Autodesk Fusion 360 part; units mm, degrees
sketch "Sketch1" plane through (0, 0, 0) normal (0, 1, 0) x (1, 0, 0)
  circle A0 centre (0, 0) radius 45
  dimension "d1" = 90
extrude "Extrude1" add sketch "Sketch1" along normal blind 70 draft -15
sketch "Sketch2" plane through (0, 0, 0) normal (0, 1, 0) x (1, 0, 0)
  circle A0 centre (0, 0) radius 42
  dimension "d4" = 84
extrude "Extrude2" cut sketch "Sketch2" along normal blind 70 draft -15
extrude "Extrude3" add 1 faces at (25.1459, 70, 1.3038) along direction (0, 1, 0) blind 35
Verification items for the finished model (mm, model axes). Coordinates: 2 decimals unless noted, no trailing zeros. Order: outer loops, then holes, each group sorted by start corner. A loop starts at its lowest first (then second) coordinate and runs counter-clockwise, first axis right, second up. Notation, with made-up numbers: (67, -24.75) -> (115, -24.75) arc R17 cw to (115, -15.75) -> close; hole circle Ø1 at (20.5, 49). An arc over 180 degrees is marked (long way). Put each result on its own line as item: value. Start each with the question number.
1. Material ranges on L1, parallel to X at y = 85, z = 0; L2, parallel to Z at x = -9, y = 56.5, recorded low to high. Write a range as [from, to].
2. Cross-section at C-C, the plane y = 75. Record the boundary of the cut face in (x, z), then the cut area to 3 significant figures.
3. Cross-section at D-D, the plane y = 25. Record the boundary of the cut face in (x, z).
4. Mould release check, pull along X, two halves, no side actions. Record for faces 1 (the cylindrical face through (-3.42, 87.26, 26.02)), 2 (the conical face through (29.253, 42.288, 9.212)), 3 (the flat face through (-15.7, 105, 17.4)): released by +X, released by -X, zero draft, split by the parting line, or undercut.
5. Cross-section at B-B, the plane x = 0. Record the boundary of the cut face in (y, z).
6. Go/stop test with flat-tipped pins: pin 1 Ø4 at (y, z) = (75, -2.5) entering from -X; pin 2 Ø5 at (x, y) = (33.5, 22.5) entering from +Z; pin 3 Ø3 at (x, y) = (22, 57.5) entering from +Z. Record where each tip stops, or that it passes through.
7. Cross-section at A-A, the plane z = 0. Record the boundary of the cut face in (x, y), then the cut area to 3 significant figures.
Computed:
1. L1: [-26.24, -23.24], [23.24, 26.24]
1. L2: [-28.47, -25.31], [25.31, 28.47]
2. outline: circle Ø52.49 at (0, 0); hole circle Ø46.49 at (0, 0)
2. area: 466 mm2
3. outline: circle Ø76.6 at (0, 0); hole circle Ø70.6 at (0, 0)
4. face 1: split by the parting line
4. face 2: undercut
4. face 3: zero draft
5. outline: (0, -45) -> (70, -26.24) -> (105, -26.24) -> (105, -23.24) -> (70, -23.24) -> (0, -42) -> close; (0, 42) -> (70, 23.24) -> (105, 23.24) -> (105, 26.24) -> (70, 26.24) -> (0, 45) -> close
6. pin 1: x = -26.24
6. pin 2: z = 23.8
6. pin 3: z = 21.45
7. outline: (-45, 0) -> (-42, 0) -> (-23.24, 70) -> (-23.24, 105) -> (-26.24, 105) -> (-26.24, 70) -> close; (23.24, 70) -> (42, 0) -> (45, 0) -> (26.24, 70) -> (26.24, 105) -> (23.24, 105) -> close
7. area: 630 mm2
